The model under review builds one solid part; all positions refer to its coordinate system, in mm. A direction names the side the tool comes from. Coordinates: 2 decimals unless noted, no trailing zeros. Write each loop counter-clockwise with the first axis right and the second up, starting at its lowest first coordinate (ties: lowest second). Pieces come first, ordered by that corner, then holes. Notation, with made-up numbers: M -12.5,53 L 19.5,53 A5 ccw 19.5,61 Z; hole C 11,1 d1. An arc over 180 degrees is marked long. Answer as CSV lines item,"result". Start each with the question number.
from build123d import *

# Parameters (mm, degrees)
F0_R     = 3
F1_DEPTH = 8
F2_R     = 2.5
F3_DEPTH = 16
F4_R     = 1.5
F5_DEPTH = 16


with BuildPart() as f1:
    # F0 (on Front) → F1 (new body)
    with BuildSketch(Plane.XZ):
        Circle(F0_R)
    extrude(amount=F1_DEPTH)

    # F2 (on Front) → F3 (join)
    with BuildSketch(Plane.XZ):
        Circle(F2_R)
    extrude(amount=F3_DEPTH)

    # F4 (on Front) → F5 (cut)
    with BuildSketch(Plane.XZ):
        Circle(F4_R)
    extrude(amount=F5_DEPTH, mode=Mode.SUBTRACT)


solid = f1.part
1) Take a section at C-C on y = -10.75. Give the boundary of the cut face in (x, z), and give its area (3 significant figures).
2) Mouldability with a two-part tool opening along Z and no side actions: class faces 1 (the flat face through (1.3, 0, -1.3)), 2 (the cylindrical face through (-0.54, -11.94, -2.44)), 3 (the cylindrical face through (-1.5, -7.89, 0.07)) as +Z half, -Z half, draft (parallel to the pull), parting line (faces both ways), or undercut.
3) Tool access review of faces 4 (the flat face through (-2, -8, 2)), 5 (the flat face through (0, -16, -2)): name each direction out of +Z, -Z, +X, -X, +Y, -Y from which nothing blocks a thin tool from reaching the whole face with its end or side.
4) Take a section at D-D on z = -2.3. Give the boundary of the cut face in (x, y), and give its area (3 significant figures).
5) Take a section at B-B on x = 0. Give the boundary of the cut face in (y, z).
6) Take a section at A-A on z = 0. Give the boundary of the cut face in (x, y).
7) To check wall thickness, follow line 1 (X direction, y = -10.25, z = 0.05); line 2 (Z direction, x = -0.1, y = -4.5). State the ranges of each line that lie inside material, in increasing order. Write a range as [from, to].
8) Clearance check with a flat-ended pin moving along its axis: pin 1 Ø1.5 at (x, y) = (2, -9) entering from +Z. State where the tip first meets the part, or that it passes through.
Results:
1,outline,"C 0,0 d5; hole C 0,0 d3"
1,area,"12.6 mm²"
2,face 1,"draft"
2,face 2,"parting line"
2,face 3,"undercut"
3,face 4,"-Y"
3,face 5,"+Z, -Z, +X, -X, -Y"
4,outline,"M -1.93,-8 L -0.98,-8 L -0.98,-16 L 0.98,-16 L 0.98,-8 L 1.93,-8 L 1.93,0 L -1.93,0 Z"
4,area,"46.5 mm²"
5,outline,"M -16,-2.5 L -8,-2.5 L -8,-3 L 0,-3 L 0,-1.5 L -16,-1.5 Z; M -16,1.5 L 0,1.5 L 0,3 L -8,3 L -8,2.5 L -16,2.5 Z"
6,outline,"M -3,-8 L -2.5,-8 L -2.5,-16 L -1.5,-16 L -1.5,0 L -3,0 Z; M 1.5,-16 L 2.5,-16 L 2.5,-8 L 3,-8 L 3,0 L 1.5,0 Z"
7,line 1,"x = [-2.5, -1.5], [1.5, 2.5]"
7,line 2,"z = [-3, -1.5], [1.5, 3]"
8,pin 1,"stops at z = 2.17"
